The model under review builds one solid part; all positions refer to its coordinate system, in mm. A direction names the side the tool comes from. Coordinates: 2 decimals unless noted, no trailing zeros. Loops run counter-clockwise (first coordinate to the right, second up) from the corner with the lowest first, then second, coordinate; pieces in that order, holes last. Notation, with made-up numbers: M 51.5,-0.75 L 62.5,-0.75 A28 cw 62.5,18.25 Z; hole C 23,-12 d11. An arc over 180 degrees is marked long. One line per item, written item: value.
Autodesk Inventor part; units mm, degrees
ref_plane "YZ Plane" through (0, 0, 0) normal (1, 0, 0) x (0, 1, 0)
ref_plane "XZ Plane" through (0, 0, 0) normal (0, 1, 0) x (-1, 0, 0)
ref_plane "XY Plane" through (0, 0, 0) normal (0, 0, 1) x (1, 0, 0)
sketch "Sketch1" plane through (0, 0, 0) normal (0, 1, 0) x (-1, 0, 0)
  circle A0 centre (0, 0) radius 25
  dimension "d0" = 50
extrude "Extrusion1" add sketch "Sketch1" along normal blind 20
fillet "Fillet1" radius 10 1 edges at (25, 20, 0)
sketch "Sketch2" plane through (0, 20, 0) normal (0, 1, 0) x (1, 0, 0)
  circle A0 centre (0, 0) radius 8.75
  dimension "d4" = 17.5
extrude "Extrusion2" cut sketch "Sketch2" against normal blind 3
sketch "Sketch3" plane through (0, 17, 0) normal (0, 1, 0) x (1, 0, 0)
  circle A0 centre (0, 0) radius 8
  dimension "d7" = 16
extrude "Extrusion3" cut sketch "Sketch3" against normal blind 2
sketch "Sketch5" plane through (0, 15, 0) normal (0, 1, 0) x (1, 0, 0)
  circle A0 centre (0, 0) radius 6
  dimension "d10" = 12
extrude "Extrusion4" add sketch "Sketch5" along normal blind 1
fillet "Fillet2" radius 2 1 edges at (-6, 16, 0)
properties part number "camera"
(1) Draft analysis for pull direction Z (two halves, no side actions). For faces 3 (the face through (-23.846, 4.93, -7.509)), 4 (the face through (-6.944, 18.521, 5.324)), 5 (the face through (0, 0, 0)), state which applies: pulls with the +Z half, pulls with the -Z half, needs draft (parallel to the pull), parting line crosses it, or undercut.
Checks:
face 3: parting line crosses it
face 4: undercut
face 5: needs draft
(2) Insertion check: pin 1 Ø1 at (x, z) = (9.5, -9) entering from -Y; pin 2 Ø1 at (x, y) = (3, 7) entering from +Z; pin 3 Ø10 at (x, z) = (19, -9) entering from +Y; pin 4 Ø4 at (x, z) = (-14.5, 9.5) entering from +Y. Each pin has a flat end and moves straight along its axis. Give the tip position at first contact, or say it passes through.
Checks:
pin 1: y = 0
pin 2: z = 24.87
pin 3: y = 19.95
pin 4: y = 19.99
(3) Add section B-B on z = 0. State the section outline as (x, y) points.
Checks:
outline: M -25,0 L 25,0 L 25,10 A10 ccw 15,20 L 8.75,20 L 8.75,17 L 8,17 L 8,15 L 6,15 A2 ccw 4.27,16 L -4.27,16 A2 ccw -6,15 L -8,15 L -8,17 L -8.75,17 L -8.75,20 L -15,20 A10 ccw -25,10 Z
(4) To check wall thickness, follow L1, parallel to Y at x = -1.5, z = -3; L2, parallel to Y at x = -0.5, z = -7.5; L3, parallel to Z at x = 0, y = 17.7. State the ranges of each line that lie inside material, in increasing order. Write a range as [from, to].
Checks:
L1: [0, 16]
L2: [0, 15]
L3: [-21.38, -8.75], [8.75, 21.38]
(5) Add section A-A on x = 0. State the section outline as (y, z) points.
Checks:
outline: M 0,-25 L 10,-25 A10 ccw 20,-15 L 20,-8.75 L 17,-8.75 L 17,-8 L 15,-8 L 15,-6 A2 ccw 16,-4.27 L 16,4.27 A2 ccw 15,6 L 15,8 L 17,8 L 17,8.75 L 20,8.75 L 20,15 A10 ccw 10,25 L 0,25 Z
(6) Tool access review of faces 1 (the face through (-6.5, 20, -6.5)), 2 (the face through (-2, 15, -6)): name each direction out of +Z, -Z, +X, -X, +Y, -Y from which nothing blocks a thin tool from reaching the whole face with its end or side.
Checks:
face 1: +Z, -Z, +X, -X, +Y
face 2: +Y
(7) Add section D-D on y = 11. State the section outline as (x, z) points.
Checks:
outline: C 0,0 d49.9
(8) Add section C-C on y = 7. State the section outline as (x, z) points, then the cut area to 3 significant figures.
Checks:
outline: C 0,0 d50
area: 1,960 mm^2
